Job drawing, mm, ordinate dimensions from the low corner. One solid piece. A direction names the side the tool comes from. Round coordinates to 2 decimals unless told otherwise and drop trailing zeros. Write item = value, one per line.
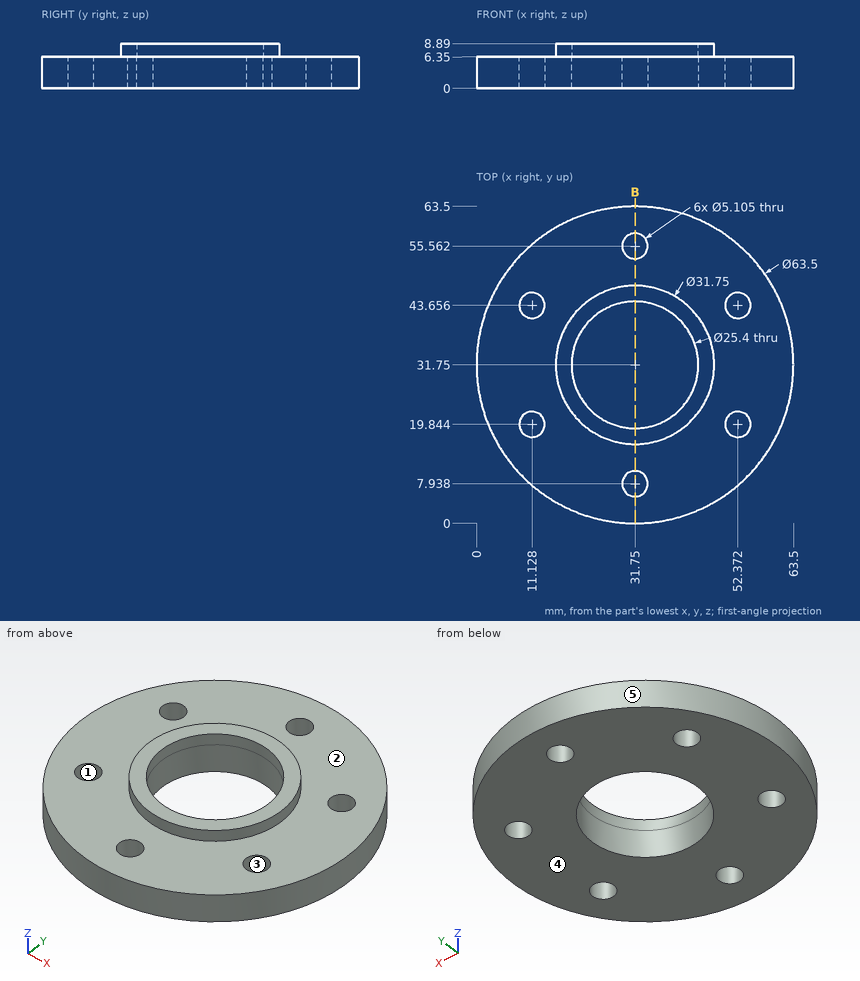
Q1. Flat gauge pins, fed straight in: pin 1 (3 mm diameter, centred on x = 22, y = 56, fed in from +Z); pin 2 (3 mm diameter, centred on y = 50.5, z = 5.5, fed in from -X) (1 decimal). Where does each tip first touch, or does it go through?
Check values:
pin_1 = 6.35
pin_2 = 5.1
Q2. Probe probe 1 along Y at (x, z) = (30.5, 1.5) (1 decimal); probe 2 along Z at (x, y) = (55.5, 20.5); probe 3 along X at (y, z) = (28, 8) (1 decimal). List the from-to ranges inside material, lowest first.
Check values:
probe_1 = 0 to 5.7, 10.2 to 19.1, 44.4 to 53.3, 57.8 to 63.5
probe_2 = 0 to 6.35
probe_3 = 16.3 to 19.6, 43.9 to 47.2
Q3. Cut at B-B, the plane x = 31.75. Give the number of separate pieces and of enclosed holes in the cut face, and give its area (3 significant figures).
Check values:
separate_pieces = 4
enclosed_holes = 0
area = 193 mm²
Q4. Mould opens along X. For the marked faces 3, 4 and 5 say: released by +X, released by -X, zero draft, split by the parting line, or undercut.
Check values:
face_3 = undercut
face_4 = zero draft
face_5 = split by the parting line
Q5. Which spindle directions (+Z, -Z, +X, -X, +Y, -Y) get a long thin tool onto all of the face, cutting with end or side? Do the marked faces 1 and 2. Say none if no direction does.
Check values:
face_1 = +Z, -Z
face_2 = +Z
